Can you work these out from the model? Positions are in its coordinate system, mm. Coordinates: 2 decimals unless noted, no trailing zeros. Order: outer loops, then holes, each group sorted by start corner. A loop starts at its lowest first (then second) coordinate and runs counter-clockwise, first axis right, second up. Notation, with made-up numbers: (79, -7.5) -> (123, -7.5) arc R23 cw to (123, 2.5) -> close; hole circle Ø1 at (62, 61.5). An arc over 180 degrees is marked (long way). Answer in a Markdown table with one row per item.
Autodesk Fusion 360 part; units mm, degrees
sketch "Sketch1" plane through (0, 0, 0) normal (0, 1, 0) x (1, 0, 0)
  circle A0 centre (0, 0) radius 15.145
  circle A1 centre (0, 17.145) radius 4
  circle A2 centre (-14.848, -8.5725) radius 4
  circle A3 centre (14.848, -8.5725) radius 4
  circle A4 centre (0, 0) radius 9
  circle A5 centre (0, 17) radius 6
  circle A6 centre (-14.7224, -8.5) radius 6
  circle A7 centre (14.7224, -8.5) radius 6
  dimension "d3" = 30.29
  dimension "d4" = 8
  dimension "d7" = 18
  dimension "d9" = 360
extrude "Extrude1" add sketch "Sketch1" along normal blind 3 contours A0 A5 A6 A7 | A0 A1 A5 | A0 A1 A5 | A0 A3 A7 | A0 A3 A7 | A0 A2 A6 | A0 A2 A6
(1) We'd pull the mould along X, two halves only. Please class faces 1 (the flat face through (-10, 3, 0)), 2 (the cylindrical face through (0.146, 1.479, 15.144)), 3 (the cylindrical face through (-13.188, 1.479, -7.446)): +X half, -X half, draft (parallel to the pull), parting line (faces both ways), or undercut.
Response values:
| item | result |
|---|---|
| face 1 | draft |
| face 2 | undercut |
| face 3 | -X half |
(2) Suppose I cut it at D-D (x = 8). Please give me the cut outline in (y, z), and give its area (3 significant figures).
Response values:
| item | result |
|---|---|
| outline | (0, -12.86) -> (3, -12.86) -> (3, -4.12) -> (0, -4.12) -> close; (0, 4.12) -> (3, 4.12) -> (3, 12.86) -> (0, 12.86) -> close |
| area | 52.4 mm2 |
(3) Suppose I cut it at C-C (z = 9.5). Please give me the cut outline in (x, y).
Response values:
| item | result |
|---|---|
| outline | (-20.64, 0) -> (-18.74, 0) -> (-18.74, 3) -> (-20.64, 3) -> close; (-10.96, 0) -> (10.96, 0) -> (10.96, 3) -> (-10.96, 3) -> close; (18.74, 0) -> (20.64, 0) -> (20.64, 3) -> (18.74, 3) -> close |
(4) Suppose I cut it at B-B (z = 0). Please give me the cut outline in (x, y) (3 decimals).
Response values:
| item | result |
|---|---|
| outline | (-15.145, 0) -> (-9, 0) -> (-9, 3) -> (-15.145, 3) -> close; (9, 0) -> (15.145, 0) -> (15.145, 3) -> (9, 3) -> close |
(5) Suppose I cut it at A-A (x = 0). Please give me the cut outline in (y, z) (3 decimals).
Response values:
| item | result |
|---|---|
| outline | (0, -23) -> (3, -23) -> (3, -21.145) -> (0, -21.145) -> close; (0, -13.145) -> (3, -13.145) -> (3, -9) -> (0, -9) -> close; (0, 9) -> (3, 9) -> (3, 15.145) -> (0, 15.145) -> close |
(6) Will these pins go through, and if not, where does the flat tip stop? pin 1 Ø1.5 at (x, y) = (-10, 0.5) entering from -Z; pin 2 Ø1.5 at (x, y) = (-14.5, 1) entering from -Z.
Response values:
| item | result |
|---|---|
| pin 1 | z = -11.99 |
| pin 2 | z = -6.35 |
(7) I need wall thicknesses on line 1 (Z direction, x = 0, y = 1.15) (3 decimals); line 2 (Z direction, x = -2, y = 1.65); line 3 (X direction, y = 2.25, z = 0) (3 decimals). Which ranges of each line are inside material? Lowest first, please. Write a range as [from, to].
Response values:
| item | result |
|---|---|
| line 1 | [-23, -21.145], [-13.145, -9], [9, 15.145] |
| line 2 | [-22.66, -20.61], [-13.68, -8.77], [8.77, 15.01] |
| line 3 | [-15.145, -9], [9, 15.145] |
